Geometry check sheet. Reference: the model listing, model coordinates, mm. A direction names the side the tool comes from. Give positions to 0.01 mm unless a question says otherwise; leave off trailing zeros. Loops run counter-clockwise (first coordinate to the right, second up) from the corner with the lowest first, then second, coordinate; pieces in that order, holes last. Notation, with made-up numbers: (30.5, -0.5) - (89.5, -0.5) arc R16 ccw to (89.5, 8.5) - close; hole circle Ø11 at (81.25, 83.5). An arc over 180 degrees is marked (long way). Use a Markdown table: item, result. Add a question column.
1. Cross-section at C-C on x = -9. Enter the section's corners in (y, z), and give its area (3 significant figures).
2. Depth check by flat-ended pin: P1, Ø4, axis at x = -2.5, z = 14, coming from the -Y side; P2, Ø1.8, axis at y = 1, z = -4.5, coming from the -X side; P3, Ø4, axis at x = 1, z = -5.5, coming from the +Y side. Enter the tip coordinate at first touch or a pass-through.
3. Cross-section at A-A on y = -15.5. Enter the section's corners in (x, z), and give its area (3 significant figures).
4. Draft check along X on faces 6 (the flat face through (-21, 25.5, 1)), 7 (the flat face through (0, 4.5, 1)), 8 (the flat face through (24, -14, 1)). Enter one of: pulls with the +X half, pulls with the -X half, needs draft (parallel to the pull), parting line crosses it, or undercut.
5. Set-up check for faces 1 (the flat face through (-4, -15, 1)), 2 (the flat face through (-22, 3, 1)), 3 (the flat face through (0, 0, -36)), 4 (the flat face through (10.902, 17.477, 0.504)), 5 (the flat face through (22, 3, 1)): record each of +Z, -Z, +X, -X, +Y, -Y from which the full face is reachable in a straight line by a thin tool's end or side.
6. Material ranges on L1, parallel to Y at x = 21, z = 11; L2, parallel to Y at x = 1.5, z = 14; L3, parallel to X at y = -17, z = -11, recorded low to high.
7. Cross-section at B-B on z = 17.5. Enter the section's corners in (x, y).
8. Cross-section at D-D on y = 13. Enter the section's corners in (x, z), and give its area (3 significant figures).
from build123d import *

# Parameters (mm, degrees)
BOSS_EXTRUDE1_DEPTH = 36
CUT_EXTRUDE1_DEPTH  = 81.06403687


with BuildPart() as part:
    # Sketch1 → Boss-Extrude1 (new, symmetric)
    with BuildSketch(Plane.XY):
        Polygon((-24, 25.5), (-4, 25.5), (-4, 4.5), (4, 4.5), (4, 25.5), (24, 25.5), (24, 3), (20, 3), (20, -3), (24, -3), (24, -25.5), (4, -25.5), (4, -12.5), (-4, -12.5), (-4, -25.5), (-24, -25.5), (-24, -3), (-20, -3), (-20, 3), (-24, 3), align=None)
    extrude(amount=BOSS_EXTRUDE1_DEPTH, both=True)

    # Sketch3 → Cut-Extrude1 (cut, through all)
    with BuildSketch(Plane.XY.offset(36)):
        Polygon((-4, 9.675878591), (-18, 25.5), (-4, 25.5), align=None)
        Polygon((4, 9.675878591), (18, 25.5), (4, 25.5), align=None)
        Polygon((4, -17.157724852), (11, -25.5), (4, -25.5), align=None)
        Polygon((-4, -17.157724852), (-11, -25.5), (-4, -25.5), align=None)
    extrude(amount=-CUT_EXTRUDE1_DEPTH, mode=Mode.SUBTRACT)


solid = part.part
Values found:
| question | item | result |
|---|---|---|
| 1 | outline | (-23.12, -36) - (15.33, -36) - (15.33, 36) - (-23.12, 36) - close |
| 1 | area | 2,770 mm2 |
| 2 | P1 | stops at y = -17.75 |
| 2 | P2 | stops at x = -20 |
| 2 | P3 | stops at y = 4.5 |
| 3 | outline | (-24, -36) - (-4, -36) - (-4, 36) - (-24, 36) - close; (4, -36) - (24, -36) - (24, 36) - (4, 36) - close |
| 3 | area | 2,880 mm2 |
| 4 | face 6 | needs draft |
| 4 | face 7 | undercut |
| 4 | face 8 | pulls with the +X half |
| 5 | face 1 | +Z, -Z, -Y |
| 5 | face 2 | +Z, -Z, -X |
| 5 | face 3 | -Z, +X, -X, +Y, -Y |
| 5 | face 4 | +Z, -Z, +Y |
| 5 | face 5 | +Z, -Z, +X |
| 6 | L1 | y = -25.5 to -3, 3 to 25.5 |
| 6 | L2 | y = -12.5 to 4.5 |
| 6 | L3 | x = -24 to -4, 4 to 24 |
| 7 | outline | (-24, -25.5) - (-11, -25.5) - (-4, -17.16) - (-4, -12.5) - (4, -12.5) - (4, -17.16) - (11, -25.5) - (24, -25.5) - (24, -3) - (20, -3) - (20, 3) - (24, 3) - (24, 25.5) - (18, 25.5) - (4, 9.68) - (4, 4.5) - (-4, 4.5) - (-4, 9.68) - (-18, 25.5) - (-24, 25.5) - (-24, 3) - (-20, 3) - (-20, -3) - (-24, -3) - close |
| 8 | outline | (-24, -36) - (-6.94, -36) - (-6.94, 36) - (-24, 36) - close; (6.94, -36) - (24, -36) - (24, 36) - (6.94, 36) - close |
| 8 | area | 2,460 mm2 |
